```python
from build123d import *

# Parameters (mm, degrees)
SKETCH1_R           = 55
BOSS_EXTRUDE1_DEPTH = 14.8
SHELL1_T            = -5
SKETCH2_R           = 35
CUT_EXTRUDE1_DEPTH  = 6
SKETCH3_R           = 42
CUT_EXTRUDE2_DEPTH  = 15.8
SKETCH4_R           = 4.15
CUT_EXTRUDE3_DEPTH  = 15.8
SKETCH6_R           = 50
CUT_EXTRUDE4_DEPTH  = 2
CUT_EXTRUDE5_DEPTH  = 4
FILLET1_R           = 10
SKETCH8_OUTSIDE_W   = 143.254
SKETCH8_OUTSIDE_H   = 143.254
SKETCH8_OUTSIDE_R   = 52.35
CUT_EXTRUDE6_DEPTH  = 4.8
CHAMFER1_SIZE       = 2
CHAMFER1_SIZE2      = 1.154700538
SKETCH9_R           = 52.5
CUT_EXTRUDE7_DEPTH  = 5


with BuildPart() as part:
    # Sketch1 → Boss-Extrude1 (new body)
    with BuildSketch(Plane(origin=(0, 0, 0), x_dir=(1, 0, 0), z_dir=(0, 1, 0))):
        with Locations(Location((0, 0, 0), (0, 0, 270))):  # turned: the seam where the file's is
            Circle(SKETCH1_R)
    extrude(amount=BOSS_EXTRUDE1_DEPTH)

    # Shell1
    shell1_openings = [part.faces().sort_by_distance(p)[0] for p in [
        (0, 0, 0),
    ]]
    offset(amount=SHELL1_T, openings=shell1_openings, kind=Kind.INTERSECTION)

    # Sketch2 → Cut-Extrude1 (cut, through all)
    with BuildSketch(Plane.XZ.offset(-9.8)):
        with Locations(Location((0, 0, 0), (0, 0, 270))):  # turned: the seam where the file's is
            Circle(SKETCH2_R)
    extrude(amount=-CUT_EXTRUDE1_DEPTH, mode=Mode.SUBTRACT)

    # Sketch3 → Cut-Extrude2 (cut, through all)
    with BuildSketch(Plane(origin=(0, 14.8, 0), x_dir=(1, 0, 0), z_dir=(0, 1, 0))):
        with Locations(Location((0, 0, 0), (0, 0, 270))):  # turned: the seam where the file's is
            Circle(SKETCH3_R)
    extrude(amount=-CUT_EXTRUDE2_DEPTH, mode=Mode.SUBTRACT)

    # Sketch4 → Cut-Extrude3 (cut, through all)
    with BuildSketch(Plane(origin=(0, 14.8, 0), x_dir=(1, 0, 0), z_dir=(0, 1, 0))):
        with Locations(Location((-33.234018716, -33.234018716, 0), (0, 0, 270))):  # turned: the seam where the file's is
            Circle(SKETCH4_R)
        with Locations(Location((-33.234018716, 33.234018716, 0), (0, 0, 270))):  # turned: the seam where the file's is
            Circle(SKETCH4_R)
        with Locations(Location((33.234018716, 33.234018716, 0), (0, 0, 270))):  # turned: the seam where the file's is
            Circle(SKETCH4_R)
        with Locations(Location((33.234018716, -33.234018716, 0), (0, 0, 270))):  # turned: the seam where the file's is
            Circle(SKETCH4_R)
    extrude(amount=-CUT_EXTRUDE3_DEPTH, mode=Mode.SUBTRACT)

    # Sketch6 → Cut-Extrude4 (cut)
    with BuildSketch(Plane.XZ.offset(-9.8)):
        Circle(SKETCH6_R)
    extrude(amount=-CUT_EXTRUDE4_DEPTH, mode=Mode.SUBTRACT)

    # Sketch7 → Cut-Extrude5 (cut, through all)
    with BuildSketch(Plane.XZ.offset(-11.8)):
        with BuildLine():
            Line((15, 33.234018716), (15, 47.696960071))
            ThreePointArc((15, 47.696960071), (0, 50), (-15, 47.696960071))
            Line((-15, 47.696960071), (-15, 33.234018716))
            Line((-15, 33.234018716), (15, 33.234018716))
        make_face()
    extrude(amount=-CUT_EXTRUDE5_DEPTH, mode=Mode.SUBTRACT)

    # Fillet1
    fillet1_edges = [part.edges().sort_by_distance(p)[0] for p in [
        (-15, 13.3, 39.230090492),
        (15, 13.3, 39.230090492),
    ]]
    fillet(fillet1_edges, radius=FILLET1_R)

    # Sketch8 outside → Cut-Extrude6 (cut)
    with BuildSketch(Plane(origin=(0, 14.8, 0), x_dir=(1, 0, 0), z_dir=(0, 1, 0))):
        Rectangle(SKETCH8_OUTSIDE_W, SKETCH8_OUTSIDE_H)
        with Locations(Location((0, 0, 0), (0, 0, 270))):  # turned: the seam where the file's is
            Circle(SKETCH8_OUTSIDE_R, mode=Mode.SUBTRACT)
    extrude(amount=-CUT_EXTRUDE6_DEPTH, mode=Mode.SUBTRACT)

    # Chamfer1
    chamfer1_edges = [part.edges().sort_by_distance(p)[0] for p in [
        (0, 14.8, -52.35),
    ]]
    chamfer1_side = [part.faces().sort_by_distance(p)[0] for p in [
        (0, 12.4, -52.35),
    ]]
    chamfer(chamfer1_edges, length=CHAMFER1_SIZE, length2=CHAMFER1_SIZE2, reference=chamfer1_side[0])

    # Sketch9 → Cut-Extrude7 (cut)
    with BuildSketch(Plane.XZ):
        with Locations(Location((0, 0, 0), (0, 0, 270))):  # turned: the seam where the file's is
            Circle(SKETCH9_R)
    extrude(amount=-CUT_EXTRUDE7_DEPTH, mode=Mode.SUBTRACT)


solid = part.part
```
CAD build for the part. Positions are in the model's coordinates, mm. A direction names the side the tool comes from. Coordinates: 2 decimals unless noted, no trailing zeros. Order: outer loops, then holes, each group sorted by start corner. A loop starts at its lowest first (then second) coordinate and runs counter-clockwise, first axis right, second up.
(1) Mould opens along Z. For faces 1 (the face through (49, 10, 20)), 2 (the face through (36.04, 11.06, -36.29)), 3 (the face through (15.725, 11.42, 49.933)) say: released by +Z, released by -Z, zero draft, split by the parting line, or undercut.
Solution:
face 1: zero draft
face 2: undercut
face 3: split by the parting line
(2) Saw through at C-C, the plane z = -35.5. Count the separate pieces of the cut face and the enclosed holes in it, and give its area (3 significant figures).
Solution:
separate pieces: 4
enclosed holes: 0
area: 144 mm2
(3) Drill centre lines: L1, parallel to X at y = 1.5, z = 0; L2, parallel to X at y = 13.5, z = 36; L3, parallel to X at y = 4.75, z = 27 (3 decimals). Where is each one in solid material? Low to high.
Solution:
L1: x = -55 to -52.5, 52.5 to 55
L2: x = -37.45 to -36.33, -30.14 to -21.63, 21.63 to 30.14, 36.33 to 37.45
L3: x = -47.917 to -45.025, 45.025 to 47.917
(4) Pin check, flat tips, straight feed: pin 1 Ø4 at (y, z) = (5, -24.5) entering from -X; pin 2 Ø1.1 at (y, z) = (14, 47) entering from +X; pin 3 Ø3 at (y, z) = (8, 6.5) entering from -X. Stop position of each tip, or through.
Solution:
pin 1: stops at x = -50.19
pin 2: stops at x = 22.81
pin 3: stops at x = -54.77
(5) Which spindle directions (+Z, -Z, +X, -X, +Y, -Y) get a long thin tool onto all of the face, cutting with end or side? Do faces 4 (the face through (-11, 11.8, -41)), 5 (the face through (4, 14.8, -42)), 6 (the face through (-16.43, 13.32, 40.44)). Say none if no direction does.
Solution:
face 4: -Y
face 5: +Z, -Z, +X, -X, +Y
face 6: +Y, -Y
(6) Saw through at A-A, the plane z = 0. Write the cut outline in (x, y), and give its area (3 significant figures).
Solution:
outline: (-55, 0) - (-52.5, 0) - (-52.5, 5) - (-50, 5) - (-50, 11.8) - (-42, 11.8) - (-42, 14.8) - (-51.2, 14.8) - (-52.35, 12.8) - (-52.35, 10) - (-55, 10) - close; (42, 11.8) - (50, 11.8) - (50, 5) - (52.5, 5) - (52.5, 0) - (55, 0) - (55, 10) - (52.35, 10) - (52.35, 12.8) - (51.2, 14.8) - (42, 14.8) - close
area: 143 mm2
(7) Saw through at B-B, the plane x = 0. Write the cut outline in (y, z), and give its area (3 significant figures).
Solution:
outline: (0, -55) - (10, -55) - (10, -52.35) - (12.8, -52.35) - (14.8, -51.2) - (14.8, -42) - (11.8, -42) - (11.8, -50) - (5, -50) - (5, -52.5) - (0, -52.5) - close; (0, 52.5) - (5, 52.5) - (5, 50) - (14.8, 50) - (14.8, 51.2) - (12.8, 52.35) - (10, 52.35) - (10, 55) - (0, 55) - close
area: 119 mm2
